from build123d import *

# Parameters (mm, degrees)
SKETCH1_W               = 120
SKETCH1_H               = 120
BOSS_EXTRUDE3_DEPTH     = 30
SKETCH5_R               = 35
BOSS_EXTRUDE5_DEPTH     = 25
CUT_EXTRUDE3_DEPTH      = 75
CUT_EXTRUDE3_DEPTH_BACK = 67
SKETCH7_R               = 25
FILLET3_R               = 10
SHELL1_T                = -2


with BuildPart() as part:
    # Sketch1 → Boss-Extrude3 (new body)
    with BuildSketch(Plane.XY):
        with Locations((60, 60)):
            Rectangle(SKETCH1_W, SKETCH1_H)
    extrude(amount=BOSS_EXTRUDE3_DEPTH)

    # Sketch5 → Boss-Extrude5 (add)
    with BuildSketch(Plane.XY):
        with Locations((60, 60)):
            Circle(SKETCH5_R)
    extrude(amount=-BOSS_EXTRUDE5_DEPTH)

    # Sketch7 → Cut-Extrude3 (cut, two sides: drawn at the far end of the back side and taken through both)
    with BuildSketch(Plane.XY.offset(-CUT_EXTRUDE3_DEPTH_BACK)):
        with Locations((60, 60)):
            Circle(SKETCH7_R)
    extrude(amount=CUT_EXTRUDE3_DEPTH + CUT_EXTRUDE3_DEPTH_BACK, mode=Mode.SUBTRACT)

    # Fillet3
    fillet3_edges = [part.edges().sort_by_distance(p)[0] for p in [
        (0, 120, 15),
        (120, 120, 15),
        (120, 0, 15),
        (0, 0, 15),
    ]]
    fillet(fillet3_edges, radius=FILLET3_R)

    # Shell1
    shell1_openings = [part.faces().sort_by_distance(p)[0] for p in [
        (60, 1.697056275, 30),
    ]]
    offset(amount=SHELL1_T, openings=shell1_openings, kind=Kind.INTERSECTION)


solid = part.part
For this review, take the finished solid that the model builds, in its own axes (mm). A direction names the side the tool comes from. Round coordinates to 2 decimals unless told otherwise and drop trailing zeros. Loops run counter-clockwise (first coordinate to the right, second up) from the corner with the lowest first, then second, coordinate; pieces in that order, holes last. Notation, with made-up numbers: (28.5, 78) - (73.5, 78) arc R27 ccw to (73.5, 94) - close; hole circle Ø2 at (26, 84.5). An arc over 180 degrees is marked (long way). Use one line per item in the form item = value.
Item 1: Consider section C-C on y = 51.5. Write out the cut boundary in (x, z), then the cut area to 3 significant figures.
Answers:
outline = (0, 0) - (26.05, 0) - (26.05, -25) - (36.49, -25) - (36.49, 30) - (34.37, 30) - (34.37, -23) - (28.11, -23) - (28.11, 2) - (2, 2) - (2, 30) - (0, 30) - close; (83.51, -25) - (93.95, -25) - (93.95, 0) - (120, 0) - (120, 30) - (118, 30) - (118, 2) - (91.89, 2) - (91.89, -23) - (85.63, -23) - (85.63, 30) - (83.51, 30) - close
area = 586 mm^2
Item 2: Tool access review of faces 4 (the cylindrical face through (55.44, 94.7, -12.32)), 5 (the flat face through (59, 120, 15)), 6 (the flat face through (85, 87, 2)): name each direction out of +Z, -Z, +X, -X, +Y, -Y from which nothing blocks a thin tool from reaching the whole face with its end or side.
Answers:
face_4 = -Z
face_5 = +Z, -Z, +X, -X, +Y
face_6 = +Z
Item 3: Consider section A-A on z = 4.5. Write out the cut boundary in (x, y), then the cut area to 3 significant figures.
Answers:
outline = (0, 10) arc R10 ccw to (10, 0) - (110, 0) arc R10 ccw to (120, 10) - (120, 110) arc R10 ccw to (110, 120) - (10, 120) arc R10 ccw to (0, 110) - close; circle Ø54 at (60, 60); hole (2, 10) arc R8 ccw to (10, 2) - (110, 2) arc R8 ccw to (118, 10) - (118, 110) arc R8 ccw to (110, 118) - (10, 118) arc R8 ccw to (2, 110) - close; hole circle Ø50 at (60, 60)
area = 1,240 mm^2
Item 4: Clearance check with flat-ended pins moving along their axes: P1, Ø1.5, axis at x = 27.5, z = -11, coming from the -Y side; P2, Ø2, axis at x = 99.5, y = 105, coming from the +Z side; P3, Ø10, axis at x = 105, y = 83, coming from the -Z side. State where each tip first meets the part, or that it passes through.
Answers:
P1 = 45.27
P2 = 2
P3 = 0
Item 5: For line 1 (Y direction, x = 60, z = -8); line 2 (Y direction, x = 60.5, z = 15) (3 decimals); line 3 (Y direction, x = 104, z = 3), list the stretches that pass through material, from the lowest coordinate up.
Answers:
line_1 = 25 to 27, 33 to 35, 85 to 87, 93 to 95
line_2 = 0 to 2, 33.005 to 35.005, 84.995 to 86.995, 118 to 120
line_3 = 0 to 2, 118 to 120
Item 6: Consider section D-D on y = 21.5. Write out the cut boundary in (x, z).
Answers:
outline = (0, 0) - (120, 0) - (120, 30) - (118, 30) - (118, 2) - (2, 2) - (2, 30) - (0, 30) - close
Item 7: Mouldability with a two-part tool opening along X and no side actions: class faces 1 (the cylindrical face through (41.574, 76.896, 2.115)), 2 (the flat face through (84, 52, 30)), 3 (the flat face through (120, 59, 15)) as +X half, -X half, draft (parallel to the pull), parting line (faces both ways), or undercut.
Answers:
face_1 = undercut
face_2 = draft
face_3 = +X half
Item 8: Consider section B-B on x = 60. Write out the cut boundary in (y, z).
Answers:
outline = (0, 0) - (25, 0) - (25, -25) - (35, -25) - (35, 30) - (33, 30) - (33, -23) - (27, -23) - (27, 2) - (2, 2) - (2, 30) - (0, 30) - close; (85, -25) - (95, -25) - (95, 0) - (120, 0) - (120, 30) - (118, 30) - (118, 2) - (93, 2) - (93, -23) - (87, -23) - (87, 30) - (85, 30) - close
